Check sheet for the modelled part. Datum: model origin and axes. Units: mm. A direction names the side the tool comes from. Give positions to 0.01 mm unless a question says otherwise; leave off trailing zeros. Write each loop counter-clockwise with the first axis right and the second up, starting at its lowest first coordinate (ties: lowest second). Pieces come first, ordered by that corner, then holes. Notation, with made-up numbers: (49.25, -31.75) -> (78.25, -31.75) arc R14 ccw to (78.25, -24.75) -> close; hole circle Ø6 at (-19, -24). An arc over 180 degrees is marked (long way). Answer as a JSON object with one key per item and string values.
from build123d import *

# Parameters (mm, degrees)
SKETCH_1_W                 = 79
SKETCH_1_H                 = 10
EXTRUDE_1_DEPTH            = 3
SKETCH_2_W                 = 13
SKETCH_2_H                 = 3
EXTRUDE_2_DEPTH            = 43.75
EXTRUDE_3_DEPTH            = 3
RIB_1_REACH                = 87.005
SKETCH_5_WALL_W            = 215.862295072
SKETCH_5_WALL_H            = 2
RIB_START                  = -2
RIB_2_DEPTH                = 2
SKETCH_8_R                 = 1.6
CUT_EXTRUDE_1_DEPTH        = 3
FILLET_1_R                 = 2.5
SKETCH_9_R                 = 1.6
CUT_EXTRUDE_5_DEPTH        = 3
CHAMFER_2_SIZE             = 2
CHAMFER_2_OF_MIRROR_1_SIZE = 2


# Read off the part's stored shape, not the designer's step: the rib step
with BuildPart() as part:
    # Sketch 1 → Extrude 1 (new body)
    with BuildSketch(Plane(origin=(0, 0, 0), x_dir=(1, 0, 0), z_dir=(0, 1, 0))):
        with Locations((39.5, 5)):
            Rectangle(SKETCH_1_W, SKETCH_1_H)
    extrude(amount=EXTRUDE_1_DEPTH)

    # Sketch 2 → Extrude 2 (add)
    with BuildSketch(Plane(origin=(0, 3, 0), x_dir=(1, 0, 0), z_dir=(0, 1, 0))):
        with Locations((20, 5.5)):
            Rectangle(SKETCH_2_W, SKETCH_2_H)
    extrude_2 = extrude(amount=EXTRUDE_2_DEPTH)

    # Sketch 4 → Extrude 3 (add)
    with BuildSketch(Plane.XY.offset(-4)):
        with BuildLine():
            Line((13.5, 46.75), (26.5, 46.75))
            ThreePointArc((26.5, 46.75), (20, 53.25), (13.5, 46.75))
        make_face()
    extrude_3 = extrude(amount=-EXTRUDE_3_DEPTH)

    # Sketch 5 wall → Rib 1 (add, up to next)
    with BuildSketch(Plane(origin=(13.5, 24.875, -8.5), x_dir=(0, 0.997657238183, 0.068410782047), z_dir=(0, 0.068410782047, -0.997657238183)), mode=Mode.PRIVATE) as rib_1_sk1:
        with Locations((0, 1)):
            Rectangle(SKETCH_5_WALL_W, SKETCH_5_WALL_H)
    rib_1_tool1 = extrude(rib_1_sk1.sketch, amount=-RIB_1_REACH, mode=Mode.PRIVATE) - part.part
    rib_1 = rib_1_tool1.solids().sort_by_distance((13.5, 24.875, -8.5))[0]
    add(rib_1)

    # Rib 2 outline → Rib 2 (add)
    with BuildSketch(Plane(origin=(26.5, 0, 0), x_dir=(0, 0, -1), z_dir=(1, 0, 0)).offset(RIB_START)):
        Polygon((10, 3), (7, 46.75), (7, 3), align=None)
    rib_2 = extrude(amount=RIB_2_DEPTH)

    # Sketch 8 → Cut-Extrude 1 (cut)
    with BuildSketch(Plane.XY.offset(-4)):
        with Locations((20, 9.75)):
            Circle(SKETCH_8_R)
        with Locations((20, 46.75)):
            Circle(SKETCH_8_R)
    cut_extrude_1 = extrude(amount=-CUT_EXTRUDE_1_DEPTH, mode=Mode.SUBTRACT)

    # Fillet 1
    fillet_1_edges = [part.edges().sort_by_distance(p)[0] for p in [
        (0, 1.5, -10),
        (79, 1.5, -10),
        (79, 1.5, 0),
        (0, 1.5, 0),
    ]]
    fillet(fillet_1_edges, radius=FILLET_1_R)

    # Sketch 9 → Cut-Extrude 5 (cut)
    with BuildSketch(Plane(origin=(0, 3, 0), x_dir=(1, 0, 0), z_dir=(0, 1, 0))):
        with Locations(Location((8, 5, 0), (0, 0, 270))):
            Circle(SKETCH_9_R)
        with Locations(Location((71, 5, 0), (0, 0, 270))):
            Circle(SKETCH_9_R)
    extrude(amount=-CUT_EXTRUDE_5_DEPTH, mode=Mode.SUBTRACT)

    # Chamfer 2
    chamfer_2_edges = [part.edges().sort_by_distance(p)[0] for p in [
        (13.5, 3, -7),
        (20, 3, -4),
        (26.5, 3, -7),
    ]]
    chamfer(chamfer_2_edges, length=CHAMFER_2_SIZE)

    # Mirror 1: Extrude 2, Extrude 3, Rib 1, Rib 2, Cut-Extrude 1 across plane
    add(extrude_2.mirror(Plane.ZY.offset(-39.5)))
    add(extrude_3.mirror(Plane.ZY.offset(-39.5)))
    add(rib_1.mirror(Plane.ZY.offset(-39.5)))
    add(rib_2.mirror(Plane.ZY.offset(-39.5)))
    add(cut_extrude_1.mirror(Plane.ZY.offset(-39.5)), mode=Mode.SUBTRACT)

    # Chamfer 2 of Mirror 1
    chamfer_2_of_mirror_1_edges = [part.edges().sort_by_distance(p)[0] for p in [
        (65.5, 3, -7),
        (59, 3, -4),
        (52.5, 3, -7),
    ]]
    chamfer(chamfer_2_of_mirror_1_edges, length=CHAMFER_2_OF_MIRROR_1_SIZE)


solid = part.part
1. Sectioned sample at D-D, the plane y = 29.5. Enter the section's corners in (x, z).
Determined:
{"outline": "(13.5, -8.18) -> (15.5, -8.18) -> (15.5, -7) -> (24.5, -7) -> (24.5, -8.18) -> (26.5, -8.18) -> (26.5, -4) -> (13.5, -4) -> close; (52.5, -8.18) -> (54.5, -8.18) -> (54.5, -7) -> (63.5, -7) -> (63.5, -8.18) -> (65.5, -8.18) -> (65.5, -4) -> (52.5, -4) -> close"}
2. Scan lines: L1, parallel to X at y = 1.05, z = -5; L2, parallel to Y at x = 20, z = -4.85; L3, parallel to X at y = 35, z = -7.5. Record each from-to range of solid material in increasing order. Write a range as [from, to].
Determined:
{"L1": "[0, 6.4], [9.6, 69.4], [72.6, 79]", "L2": "[0, 8.15], [11.35, 45.15], [48.35, 53.25]", "L3": "[13.5, 15.5], [24.5, 26.5], [52.5, 54.5], [63.5, 65.5]"}
3. Go/stop test with flat-tipped pins: P1, Ø10, axis at x = 14, y = 12.5, coming from the +Z side; P2, Ø5, axis at y = 15.5, z = -6, coming from the +X side; P3, Ø1.5, axis at y = 31.5, z = -8.5, coming from the -X side. Record where each tip stops, or that it passes through.
Determined:
{"P1": "z = -4", "P2": "x = 65.5", "P3": "x = 13.5"}
4. Mould release check, pull along X, two halves, no side actions. Record for faces 6 (the face through (51.5, 4, -6.9)), 7 (the face through (39, 1, -10)), 8 (the face through (13.5, 26, -6)): released by +X, released by -X, zero draft, split by the parting line, or undercut.
Determined:
{"face 6": "undercut", "face 7": "zero draft", "face 8": "released by -X"}
5. Sectioned sample at C-C, the plane x = 59. Enter the section's corners in (y, z), plus the area to 3 significant figures.
Determined:
{"outline": "(0, -10) -> (3, -10) -> (3, -7) -> (8.15, -7) -> (8.15, -4) -> (5, -4) -> (3, -2) -> (3, 0) -> (0, 0) -> close; (11.35, -7) -> (45.15, -7) -> (45.15, -4) -> (11.35, -4) -> close; (48.35, -7) -> (53.25, -7) -> (53.25, -4) -> (48.35, -4) -> close", "area": "164 mm^2"}
6. Access from +Z, -Z, +X, -X, +Y, -Y to the whole of each face (thin tool, end or side, straight path). Record for faces 1 (the face through (26.5, 26, -6)), 2 (the face through (39, 0, -5)), 3 (the face through (59, 29, -4)), 4 (the face through (57.52, 46.14, -5.48)), 5 (the face through (59, 3, -9)).
Determined:
{"face 1": "+Z, -Z, +Y", "face 2": "+Z, -Z, +X, -X, -Y", "face 3": "+Z, +X, -X, +Y", "face 4": "+Z, -Z", "face 5": "-Z, +Y"}
7. Sectioned sample at A-A, the plane x = 71. Enter the section's corners in (y, z).
Determined:
{"outline": "(0, -10) -> (3, -10) -> (3, -6.6) -> (0, -6.6) -> close; (0, -3.4) -> (3, -3.4) -> (3, 0) -> (0, 0) -> close"}
8. Sectioned sample at B-B, the plane y = 9.75. Enter the section's corners in (x, z).
Determined:
{"outline": "(13.5, -9.54) -> (15.5, -9.54) -> (15.5, -7) -> (18.4, -7) -> (18.4, -4) -> (13.5, -4) -> close; (21.6, -7) -> (24.5, -7) -> (24.5, -9.54) -> (26.5, -9.54) -> (26.5, -4) -> (21.6, -4) -> close; (52.5, -9.54) -> (54.5, -9.54) -> (54.5, -7) -> (57.4, -7) -> (57.4, -4) -> (52.5, -4) -> close; (60.6, -7) -> (63.5, -7) -> (63.5, -9.54) -> (65.5, -9.54) -> (65.5, -4) -> (60.6, -4) -> close"}
